from build123d import *

# Parameters (mm, degrees)
F1_DEPTH      = 57.15
F3_DEPTH      = 2.54
F4_R          = 12.699236
F5_DEPTH      = 98.806
F5_DEPTH_BACK = 38.1
F6_R          = 1.785731
F6_R_2        = 1.796868
F7_DEPTH      = 49.53


with BuildPart() as f1:
    # F0 (on Front) → F1 (new body, symmetric)
    with BuildSketch(Plane.XZ):
        Polygon((-38.091652, 0), (0, 0), (38.091652, 0), (27.730556, 25.96328), (0, 25.96328), (-27.730556, 25.96328), align=None)
    extrude(amount=F1_DEPTH, both=True)

    # F2 (on Top) → F3 (join, symmetric)
    with BuildSketch(Plane.XY):
        Polygon((-41.44403, 58.712374), (-41.44403, 0), (-41.44403, -58.712374), (0, -58.712374), (41.44403, -58.712374), (41.44403, 0), (41.44403, 58.712374), (0, 58.712374), align=None)
    extrude(amount=F3_DEPTH, both=True)

    # F4 (on Front) → F5 (cut, two sides)
    with BuildSketch(Plane.XZ) as f5_sk:
        with Locations((0, 12.640108)):
            Circle(F4_R)
    extrude(amount=F5_DEPTH, mode=Mode.SUBTRACT)
    extrude(f5_sk.sketch, amount=-F5_DEPTH_BACK, mode=Mode.SUBTRACT)

    # F6 (on Right) → F7 (cut, symmetric)
    with BuildSketch(Plane.YZ):
        with Locations((-44.18141, 0)):
            Circle(F6_R)
        with Locations((45.368254, 0)):
            Circle(F6_R_2)
    extrude(amount=F7_DEPTH, both=True, mode=Mode.SUBTRACT)


solid = f1.part
Source: CAD feature listing. Evaluate the final solid. Frame: model axes, mm. A direction names the side the tool comes from. Round coordinates to 2 decimals unless told otherwise and drop trailing zeros. Loops run counter-clockwise (first coordinate to the right, second up) from the corner with the lowest first, then second, coordinate; pieces in that order, holes last.
Q1. Section D-D, the plane y = -44. Return loops of the section in (x, z).
Q2. Section B-B, the plane y = 13. Return loops of the section in (x, z), plus the area to 3 significant figures.
Q3. Ray query, line 1 (Z direction, x = 0, y = -11); line 2 (Y direction, x = 14, z = 24.25); line 3 (X direction, y = -29.5, z = 16.25). Return the intervals inside material, ascending.
Q4. Section C-C, the plane z = 4.25. Return loops of the section in (x, y).
Q5. Access query for faces 5 (the face through (-1, 57.15, 14)), 6 (the face through (-1.65, -9.63, 25.23)), 7 (the face through (-9, -57.15, 22)). Directions: +Z, -Z, +X, -X, +Y, -Y. A direction counts if a zero-diameter tool reaches every point of the face in a straight line with its end or side. Return the directions, or none.
Q6. Mould query, pull axis Y, two halves, no side actions, for faces 1 (the face through (0, -1, 25.963)), 2 (the face through (0.58, 43.573, 0.079)), 3 (the face through (1, 58.712, 0)), 4 (the face through (0, 38.1, 13)). Classes: pulls with the +Y half, pulls with the -Y half, needs draft (parallel to the pull), parting line crosses it, or undercut.
Q7. First-contact query: P1, Ø4, axis at y = -14, z = 20.5, coming from the +X side; P2, Ø12, axis at y = -11, z = 18, coming from the +X side; P3, Ø12, axis at y = 22.5, z = 11, coming from the -X side. Flat tips, straight axial feed; report the tip coordinate or a pass-through.
Q8. Section A-A, the plane x = 25.5. Return loops of the section in (y, z).
Solutions:
1. outline: (-41.44, -2.54) - (41.44, -2.54) - (41.44, -1.78) - (-41.44, -1.78) - close; (-41.44, 1.78) - (-6.58, 1.78) arc R12.7 cw (long way) to (6.58, 1.78) - (41.44, 1.78) - (41.44, 2.54) - (37.08, 2.54) - (27.73, 25.96) - (-27.73, 25.96) - (-37.08, 2.54) - (-41.44, 2.54) - close
2. outline: (-41.44, -2.54) - (41.44, -2.54) - (41.44, 2.54) - (37.08, 2.54) - (27.73, 25.96) - (-27.73, 25.96) - (-37.08, 2.54) - (-41.44, 2.54) - close; hole circle Ø25.4 at (0, 12.64)
2. area: 1,430 mm2
3. line 1: z = -2.54 to -0.06, 25.34 to 25.96
3. line 2: y = -57.15 to 57.15
3. line 3: x = -31.61 to -12.18, 12.18 to 31.61
4. outline: (-36.4, -57.15) - (-9.53, -57.15) - (-9.53, 38.1) - (9.53, 38.1) - (9.53, -57.15) - (36.4, -57.15) - (36.4, 57.15) - (-36.4, 57.15) - close
5. face 5: +Z, +X, -X, +Y
5. face 6: -Y
5. face 7: +Z, +X, -X, -Y
6. face 1: needs draft
6. face 2: undercut
6. face 3: pulls with the +Y half
6. face 4: pulls with the -Y half
7. P1: stops at x = 30.71
7. P2: stops at x = 33.3
7. P3: stops at x = -36.1
8. outline: (-58.71, -2.54) - (58.71, -2.54) - (58.71, 2.54) - (57.15, 2.54) - (57.15, 25.96) - (-57.15, 25.96) - (-57.15, 2.54) - (-58.71, 2.54) - close; hole circle Ø3.57 at (-44.18, 0); hole circle Ø3.59 at (45.37, 0)
